Can you work these out from the model? Positions are in its coordinate system, mm. Face numbers are marked on the shaded views. Coordinates: 2 decimals unless noted, no trailing zeros. Order: outer loops, then holes, each group sorted by start corner. A loop starts at its lowest first (then second) coordinate and runs counter-clockwise, first axis right, second up.
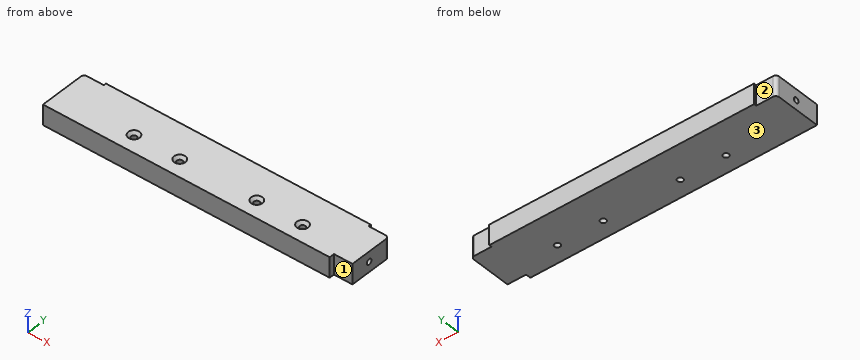
```python
from build123d import *

# Parameters (mm, degrees)
ESBO_O1_W                                      = 119
ESBO_O1_H                                      = 30
RESSALTO_EXTRUS_O1_DEPTH                       = 12
ESCAREADO_PARA_SFHCS_M31_D                     = 3.4
ESCAREADO_PARA_SFHCS_M31_CSINK_D               = 6.72
ESCAREADO_PARA_SFHCS_M31_CSINK_ANGLE           = 90
ESBO_O6_W                                      = 36.2
ESBO_O6_H                                      = 30
RESSALTO_EXTRUS_O2_DEPTH                       = 12
ESBO_O7_W                                      = 26.2
ESBO_O7_H                                      = 30
RESSALTO_EXTRUS_O3_DEPTH                       = 12
ESBO_O8_W                                      = 12
ESBO_O8_H                                      = 12
CORTE_EXTRUS_O1_DEPTH                          = 1.5
FILETE1_R                                      = 2
ESBO_O9_W                                      = 11
ESBO_O9_H                                      = 12
CORTE_EXTRUS_O2_DEPTH                          = 3
BROCA_DE_ROSQUEAR_PARA_TARRAXA_DE_M4X0_7_D     = 3.3
BROCA_DE_ROSQUEAR_PARA_TARRAXA_DE_M4X0_7_DEPTH = 10
BROCA_DE_ROSQUEAR_PARA_TARRAXA_DE_M4X0_7_TIP   = 0.991420021
ESBO_O12_W                                     = 12
ESBO_O12_H                                     = 12
CORTE_EXTRUS_O3_DEPTH                          = 1.5
FILETE2_R                                      = 2
BROCA_DE_ROSQUEAR_PARA_TARRAXA_DE_M4_2_D       = 3.3
BROCA_DE_ROSQUEAR_PARA_TARRAXA_DE_M4_2_DEPTH   = 10
BROCA_DE_ROSQUEAR_PARA_TARRAXA_DE_M4_2_TIP     = 0.991420021


with BuildPart() as part:
    # Esboço1 → Ressalto-extrusão1 (new body)
    with BuildSketch(Plane.XY):
        with Locations((-14.240307174, 185)):
            Rectangle(ESBO_O1_W, ESBO_O1_H)
    extrude(amount=RESSALTO_EXTRUS_O1_DEPTH)

    # Escareado para SFHCS M31 (through all)
    with Locations(Plane.XY.offset(12)):
        with Locations((35.859692826, 180), (-64.340307174, 180), (-37.140307174, 180), (8.659692826, 180)):
            CounterSinkHole(ESCAREADO_PARA_SFHCS_M31_D / 2, ESCAREADO_PARA_SFHCS_M31_CSINK_D / 2, counter_sink_angle=ESCAREADO_PARA_SFHCS_M31_CSINK_ANGLE)

    # Esboço6 → Ressalto-extrusão2 (add)
    with BuildSketch(Plane.XY):
        with Locations((-91.840307174, 185)):
            Rectangle(ESBO_O6_W, ESBO_O6_H)
    extrude(amount=RESSALTO_EXTRUS_O2_DEPTH)

    # Esboço7 → Ressalto-extrusão3 (add)
    with BuildSketch(Plane.XY):
        with Locations((58.359692826, 185)):
            Rectangle(ESBO_O7_W, ESBO_O7_H)
    extrude(amount=RESSALTO_EXTRUS_O3_DEPTH)

    # Esboço8 → Corte-extrusão1 (cut)
    with BuildSketch(Plane(origin=(0, 200, 0), x_dir=(1, 0, 0), z_dir=(0, 1, 0))):
        with Locations((65.459692826, -6)):
            Rectangle(ESBO_O8_W, ESBO_O8_H)
    extrude(amount=-CORTE_EXTRUS_O1_DEPTH, mode=Mode.SUBTRACT)

    # Filete1
    filete1_edges = [part.edges().sort_by_distance(p)[0] for p in [
        (71.459692826, 198.5, 6),
    ]]
    fillet(filete1_edges, radius=FILETE1_R)

    # Esboço9 → Corte-extrusão2 (cut)
    with BuildSketch(Plane.XZ.offset(-170)):
        with Locations((65.959692826, 6)):
            Rectangle(ESBO_O9_W, ESBO_O9_H)
    extrude(amount=-CORTE_EXTRUS_O2_DEPTH, mode=Mode.SUBTRACT)

    # Broca de rosquear para tarraxa de M4x0.7
    with Locations(Plane(origin=(71.459692826, 0, 0), x_dir=(0, 0, -1), z_dir=(1, 0, 0))):
        with Locations((-6, 184.75)):
            Hole(BROCA_DE_ROSQUEAR_PARA_TARRAXA_DE_M4X0_7_D / 2, depth=BROCA_DE_ROSQUEAR_PARA_TARRAXA_DE_M4X0_7_DEPTH)
            with Locations((0, 0, -(BROCA_DE_ROSQUEAR_PARA_TARRAXA_DE_M4X0_7_DEPTH + BROCA_DE_ROSQUEAR_PARA_TARRAXA_DE_M4X0_7_TIP / 2))):  # 118° drill point
                Cone(0, BROCA_DE_ROSQUEAR_PARA_TARRAXA_DE_M4X0_7_D / 2, BROCA_DE_ROSQUEAR_PARA_TARRAXA_DE_M4X0_7_TIP, mode=Mode.SUBTRACT)

    # Esboço12 → Corte-extrusão3 (cut)
    with BuildSketch(Plane(origin=(0, 200, 0), x_dir=(-1, 0, 0), z_dir=(0, 1, 0))):
        with Locations((103.940307174, 6)):
            Rectangle(ESBO_O12_W, ESBO_O12_H)
    extrude(amount=-CORTE_EXTRUS_O3_DEPTH, mode=Mode.SUBTRACT)

    # Filete2
    filete2_edges = [part.edges().sort_by_distance(p)[0] for p in [
        (-109.940307174, 198.5, 6),
    ]]
    fillet(filete2_edges, radius=FILETE2_R)

    # Broca de rosquear para tarraxa de M4 2
    with Locations(Plane.ZY.offset(109.940307174)):
        with Locations((5.5, 184.558440573), (-130.6, 184.75)):
            Hole(BROCA_DE_ROSQUEAR_PARA_TARRAXA_DE_M4_2_D / 2, depth=BROCA_DE_ROSQUEAR_PARA_TARRAXA_DE_M4_2_DEPTH)
            with Locations((0, 0, -(BROCA_DE_ROSQUEAR_PARA_TARRAXA_DE_M4_2_DEPTH + BROCA_DE_ROSQUEAR_PARA_TARRAXA_DE_M4_2_TIP / 2))):  # 118° drill point
                Cone(0, BROCA_DE_ROSQUEAR_PARA_TARRAXA_DE_M4_2_D / 2, BROCA_DE_ROSQUEAR_PARA_TARRAXA_DE_M4_2_TIP, mode=Mode.SUBTRACT)


solid = part.part
```
1. Imagine slicing it at A-A on y = 180. Please give me the cut outline in (x, z).
Completed:
outline: (-109.94, 0) - (-66.04, 0) - (-66.04, 10.34) - (-67.7, 12) - (-109.94, 12) - close; (-62.64, 0) - (-38.84, 0) - (-38.84, 10.34) - (-40.5, 12) - (-60.98, 12) - (-62.64, 10.34) - close; (-35.44, 0) - (6.96, 0) - (6.96, 10.34) - (5.3, 12) - (-33.78, 12) - (-35.44, 10.34) - close; (10.36, 0) - (34.16, 0) - (34.16, 10.34) - (32.5, 12) - (12.02, 12) - (10.36, 10.34) - close; (37.56, 0) - (71.46, 0) - (71.46, 12) - (39.22, 12) - (37.56, 10.34) - close
2. I'm going to push flat-ended pins straight in: pin 1 (2.5 mm diameter, centred on x = 35.86, y = 180, fed in from -Z); pin 2 (5 mm diameter, centred on x = -103, z = 7.5, fed in from +Y); pin 3 (5.5 mm diameter, centred on x = 63.5, z = 3.5, fed in from -Y); pin 4 (3.5 mm diameter, centred on y = 171, z = 3.5, fed in from +X). Where does each tip first touch, or does it pass through?
Completed:
pin 1: passes through
pin 2: stops at y = 198.5
pin 3: stops at y = 173
pin 4: stops at x = 60.46
3. Thinking about a two-plate mould opening in Y: for the marked faces 1, 2 and 3, which applies, pulls with the +Y half, pulls with the -Y half, needs draft (parallel to the pull), parting line crosses it, or undercut?
Completed:
face 1: pulls with the -Y half
face 2: pulls with the +Y half
face 3: needs draft
4. Please list where these lines run through material, in increasing order: probe 1 along X at (y, z) = (180, 6.25); probe 2 along Y at (x, z) = (-107, 5.5); probe 3 along Y at (x, z) = (67, 6).
Completed:
probe 1: x = -109.94 to -66.04, -62.64 to -38.84, -35.44 to 6.96, 10.36 to 34.16, 37.56 to 71.46
probe 2: y = 170 to 182.91, 186.21 to 198.5
probe 3: y = 173 to 183.1, 186.4 to 198.5
